Verification items for the finished model (mm, model axes). A direction names the side the tool comes from. Round coordinates to 2 decimals unless told otherwise and drop trailing zeros. Order: outer loops, then holes, each group sorted by start corner. A loop starts at its lowest first (then second) coordinate and runs counter-clockwise, first axis right, second up. Notation, with made-up numbers: M 0,-33.75 L 13,-33.75 A24 ccw 13,-16.75 Z; hole C 43.25,62 d10. An arc over 180 degrees is marked long. Return JSON: item names as keys, results as strings. Group by question number.
from build123d import *

# Parameters (mm, degrees)
SKETCH1_W           = 10
SKETCH1_H           = 30
BOSS_EXTRUDE1_DEPTH = 1
BOSS_EXTRUDE2_DEPTH = 10
FILLET1_R           = 1


with BuildPart() as part:
    # Sketch1 → Boss-Extrude1 (new body)
    with BuildSketch(Plane.XY):
        Rectangle(SKETCH1_W, SKETCH1_H)
    extrude(amount=BOSS_EXTRUDE1_DEPTH)

    # Sketch3 → Boss-Extrude2 (add, symmetric)
    with BuildSketch(Plane.XZ):
        with BuildLine():
            Line((-3.8, 1), (-3.8, 4.371779789))
            Line((-3.8, 4.371779789), (-3.072059531, 6.371779789))
            Line((-3.072059531, 6.371779789), (-2.6, 6.371779789))
            Line((-2.6, 6.371779789), (-2.6, 4.871779789))
            ThreePointArc((-2.6, 4.871779789), (-0.8, 2), (1, 4.871779789))
            Line((1, 4.871779789), (1, 6.371779789))
            Line((1, 6.371779789), (1.472059531, 6.371779789))
            Line((1.472059531, 6.371779789), (2.2, 4.371779789))
            Line((2.2, 4.371779789), (2.2, 1))
            Line((2.2, 1), (-3.8, 1))
        make_face()
    extrude(amount=BOSS_EXTRUDE2_DEPTH, both=True)

    # Fillet1
    fillet1_edges = [part.edges().sort_by_distance(p)[0] for p in [
        (-5, 15, 0.5),
        (5, 15, 0.5),
        (5, -15, 0.5),
        (-5, -15, 0.5),
    ]]
    fillet(fillet1_edges, radius=FILLET1_R)


solid = part.part
1. Cross-section at D-D (x = -2). Enter the section's corners in (y, z).
2. Cross-section at C-C (y = 8.5). Enter the section's corners in (x, z), plus the area to 3 significant figures.
3. Thickness scan on line 1 along X through (y, z) = (0.5, 4); line 2 along Z through (x, y) = (-0.8, -1.25); line 3 along Z through (x, y) = (1, 13). Record the ranges inside material, lowest first. Write a range as from..to.
4. Access from +Z, -Z, +X, -X, +Y, -Y to the whole of each face (thin tool, end or side, straight path). Record for faces 1 (the face through (1, 0, 6)), 2 (the face through (-3.8, 0, 3)), 3 (the face through (2.2, 0, 3)).
5. Draft check along X on faces 4 (the face through (-3.44, -0.14, 5.36)), 5 (the face through (0, -10, 2)), 6 (the face through (4.699, 14.715, 0.507)), 7 (the face through (-2.6, 0, 6)). Enter one of: +X half, -X half, draft (parallel to the pull), parting line (faces both ways), or undercut.
6. Go/stop test with flat-tipped pins: pin 1 (2.5 mm diameter, centred on x = -0.5, z = 2.5, fed in from +Y); pin 2 (1.7 mm diameter, centred on y = -0.5, z = 3, fed in from -X); pin 3 (3.5 mm diameter, centred on y = 4.5, z = 3, fed in from +X); pin 4 (2 mm diameter, centred on y = -11.5, z = 3.5, fed in from +X). Record where each tip stops, or that it passes through.
7. Cross-section at B-B (x = -0.8). Enter the section's corners in (y, z).
8. Cross-section at A-A (z = 4). Enter the section's corners in (x, y).
Computed:
{
 "1": {"outline": "M -15,0 L 15,0 L 15,1 L 10,1 L 10,2.4 L -10,2.4 L -10,1 L -15,1 Z"},
 "2": {"outline": "M -5,0 L 5,0 L 5,1 L 2.2,1 L 2.2,4.37 L 1.47,6.37 L 1,6.37 L 1,4.87 A2 cw long -2.6,4.87 L -2.6,6.37 L -3.07,6.37 L -3.8,4.37 L -3.8,1 L -5,1 Z", "area": "25.7 mm²"},
 "3": {"line 1": "x = -3.8..-2.8, 1.2..2.2", "line 2": "z = 0..2", "line 3": "z = 0..1"},
 "4": {"face 1": "+Z, +Y, -Y", "face 2": "+Z, -X, +Y, -Y", "face 3": "+Z, +X, +Y, -Y"},
 "5": {"face 4": "-X half", "face 5": "draft", "face 6": "+X half", "face 7": "undercut"},
 "6": {"pin 1": "stops at y = 10", "pin 2": "stops at x = -3.8", "pin 3": "stops at x = 2.2", "pin 4": "passes through"},
 "7": {"outline": "M -15,0 L 15,0 L 15,1 L 10,1 L 10,2 L -10,2 L -10,1 L -15,1 Z"},
 "8": {"outline": "M -3.8,-10 L -2.8,-10 L -2.8,10 L -3.8,10 Z; M 1.2,-10 L 2.2,-10 L 2.2,10 L 1.2,10 Z"}
}
